Print and shaded views of the part. All mm, measured from the part's lowest x, y and z. A direction names the side the tool comes from. Round coordinates to 2 decimals unless told otherwise and drop trailing zeros. Order: outer loops, then holes, each group sorted by start corner. A loop starts at its lowest first (then second) coordinate and runs counter-clockwise, first axis right, second up. Notation, with made-up numbers: M -22.5,4 L 29.5,4 A34 cw 29.5,40 Z; hole C -39.5,-28.5 d4. An arc over 180 degrees is marked long. Write each question's results on one line, items separated by ' | '. Start each with the question number.
1. Probe L1, parallel to Z at x = 7.62, y = 6.5 (1 decimal); L2, parallel to Y at x = 14.75, z = 24.5; L3, parallel to X at y = 1, z = 6 (1 decimal). List the from-to ranges inside material, lowest first. Write a range as [from, to].
2. Which spindle directions (+Z, -Z, +X, -X, +Y, -Y) get a long thin tool onto all of the face, cutting with end or side? Do the marked faces 1 and 2. Say none if no direction does.
3. Drop flat-ended pins along their axis: pin 1 Ø2.5 at (x, z) = (7.62, 6.35) entering from +Y; pin 2 Ø5 at (y, z) = (5.5, 38) entering from +X. Give the stop position or say it passes through.
4. Band-saw the part on C-C, the plane x = 10. List the corners of the cut face in (y, z) (1 decimal).
5. Band-saw the part on D-D, the plane x = 6.5. List the corners of the cut face in (y, z) (1 decimal).
6. Band-saw the part on A-A, the plane z = 6.35. List the corners of the cut face in (x, y) (1 decimal).
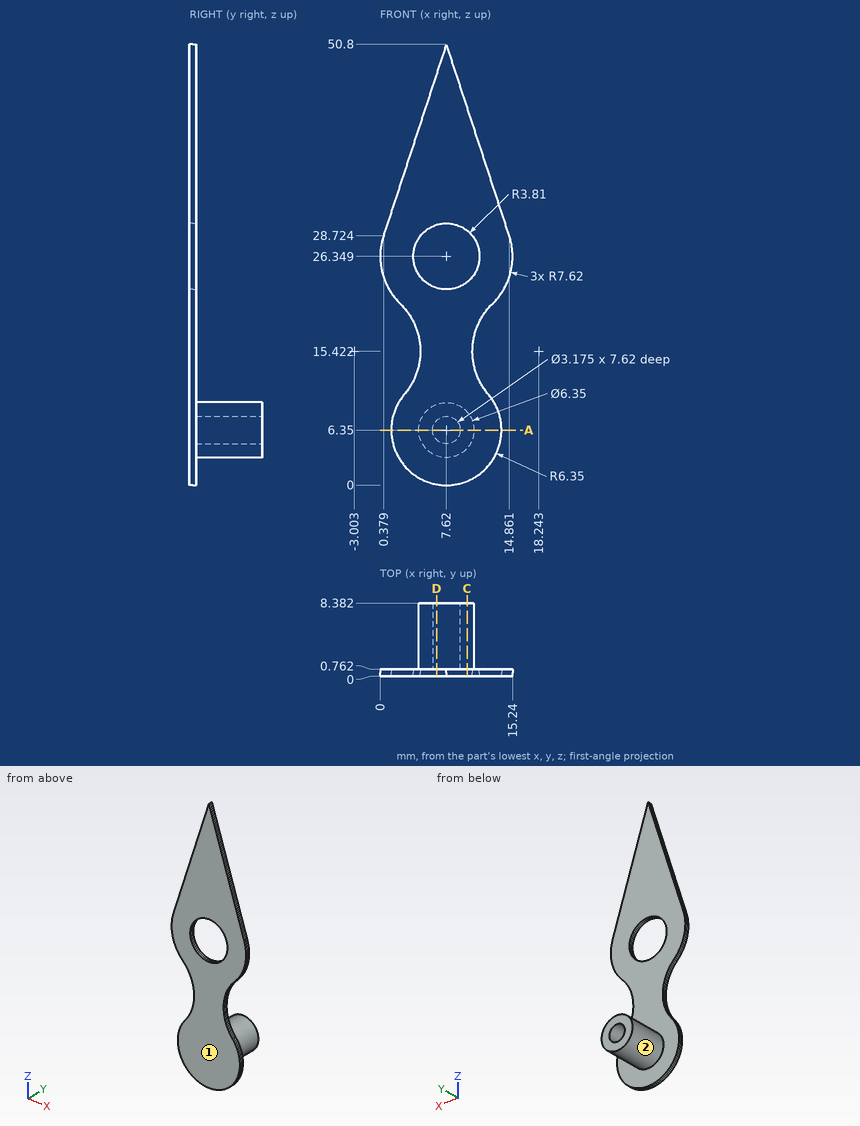
Solution:
1) L1: [3.2, 4.8], [7.9, 9.5] | L2: [0, 0.76] | L3: [4.5, 6.1], [9.2, 10.8]
2) face 1: +Z, -Z, +X, -X, -Y | face 2: +Y
3) pin 1: y = 0.76 | pin 2: through
4) outline: M 0,0.5 L 0.8,0.5 L 0.8,4.2 L 8.4,4.2 L 8.4,8.5 L 0.8,8.5 L 0.8,23.4 L 0,23.4 Z; M 0,29.3 L 0.8,29.3 L 0.8,43.5 L 0,43.5 Z
5) outline: M 0,0.1 L 0.8,0.1 L 0.8,3.4 L 8.4,3.4 L 8.4,5.2 L 0.8,5.2 L 0.8,7.5 L 8.4,7.5 L 8.4,9.3 L 0.8,9.3 L 0.8,22.7 L 0,22.7 Z; M 0,30 L 0.8,30 L 0.8,47.4 L 0,47.4 Z
6) outline: M 1.3,0 L 14,0 L 14,0.8 L 10.8,0.8 L 10.8,8.4 L 9.2,8.4 L 9.2,0.8 L 6,0.8 L 6,8.4 L 4.4,8.4 L 4.4,0.8 L 1.3,0.8 Z
